Geometry: final body of the model. Coordinates: model frame, mm. A direction names the side the tool comes from. Coordinates: 2 decimals unless noted, no trailing zeros. Write each loop counter-clockwise with the first axis right and the second up, starting at its lowest first coordinate (ties: lowest second). Pieces come first, ordered by that corner, then holes. Notation, with made-up numbers: M -2.5,13.25 L 1.5,13.25 A21 cw 1.5,48.25 Z; hole C 49,30.25 d7. An arc over 180 degrees is marked long. Write item = value, one per line. Start each with the question number.
Item 1: Section C-C on x = 15.5. Output: boundary loops of the cut face in (y, z) (1 decimal).
Item 2: Section A-A on x = 0. Output: boundary loops of the cut face in (y, z).
Item 3: Pull-direction query (Y, two-part tool) for faces 1 (the cylindrical face through (19.492, 1.086, 0.236)), 2 (the flat face through (17, 16, 12.763)), 3 (the cylindrical face through (-19.55, 21.2, 19.49)); classes: +Y half, -Y half, draft (parallel to the pull), parting line (faces both ways), or undercut.
Item 4: First-contact query: pin 1 Ø2.5 at (x, z) = (1.5, 17) entering from +Y; pin 2 Ø13 at (x, z) = (-0.5, -1.5) entering from +Y. Flat tips, straight axial feed; report the tip coordinate or a pass-through.
Item 5: Section D-D on y = 7.5. Output: boundary loops of the cut face in (x, z), plus the area to 3 significant figures.
Item 6: Section B-B on z = 0. Output: boundary loops of the cut face in (x, y).
Item 7: Ray query, L1, parallel to Z at x = -16.5, y = 27; L2, parallel to X at y = 20, z = -14.5; L3, parallel to Z at x = 0, y = 1.95. Return the intervals inside material, ascending. Write a range as [from, to].
Item 8: Reachability of faces 4 (the cylindrical face through (-19.492, 1.086, -0.236)), 5 (the cylindrical face through (17.6, 35.9, -10.2)), 6 (the flat face through (0, 12.7, 17)) from +Z, -Z, +X, -X, +Y, -Y: full face, straight path, thin tool, end or side. Return the list, or none.
from build123d import *

# Parameters (mm, degrees)
SKETCH1_W           = 26.035
SKETCH1_H           = 26.035
SKETCH1_R           = 1.778
BOSS_EXTRUDE1_DEPTH = 5.08
SKETCH9_W           = 41.275
SKETCH9_H           = 41.275
SKETCH9_W_2         = 26.035
SKETCH9_H_2         = 26.035
BOSS_EXTRUDE7_DEPTH = 38.1
CUT_EXTRUDE4_DEPTH  = 42.275
SKETCH11_R          = 3.048
CUT_EXTRUDE5_DEPTH  = 42.275
FILLET1_R           = 3.81
FILLET2_R           = 3.81
SKETCH12_R          = 5.461
SKETCH12_R_2        = 3.048
CUT_EXTRUDE6_DEPTH  = 6.096
CUT_EXTRUDE7_START  = -41.275
SKETCH12_3_R        = 5.461
CUT_EXTRUDE7_DEPTH  = 6.096
SKETCH13_W          = 25.4
SKETCH13_H          = 12.7
CUT_EXTRUDE8_DEPTH  = 42.275
FILLET3_R           = 3.81
FILLET4_R           = 3.81


with BuildPart() as part:
    # Sketch1 → Boss-Extrude1 (new body)
    with BuildSketch(Plane(origin=(0, 0, 0), x_dir=(1, 0, 0), z_dir=(0, 1, 0))):
        Rectangle(SKETCH1_W, SKETCH1_H)
        with Locations((0, 9.525)):
            Circle(SKETCH1_R, mode=Mode.SUBTRACT)
        with Locations((-9.525, 0)):
            Circle(SKETCH1_R, mode=Mode.SUBTRACT)
        with Locations((9.525, 0)):
            Circle(SKETCH1_R, mode=Mode.SUBTRACT)
        with Locations((0, -9.525)):
            Circle(SKETCH1_R, mode=Mode.SUBTRACT)
    extrude(amount=BOSS_EXTRUDE1_DEPTH)

    # Sketch9 → Boss-Extrude7 (add)
    with BuildSketch(Plane.XZ):
        Rectangle(SKETCH9_W, SKETCH9_H)
        Rectangle(SKETCH9_W_2, SKETCH9_H_2, mode=Mode.SUBTRACT)
    extrude(amount=-BOSS_EXTRUDE7_DEPTH)

    # Sketch10 → Cut-Extrude4 (cut, through all)
    with BuildSketch(Plane.XY.offset(20.6375)):
        with BuildLine():
            Line((-13.0175, 20.32), (-13.0175, 38.1))
            Line((-13.0175, 38.1), (13.0175, 38.1))
            Line((13.0175, 38.1), (13.0175, 20.32))
            ThreePointArc((13.0175, 20.32), (10.785653673, 14.931846327), (5.3975, 12.7))
            Line((5.3975, 12.7), (-5.3975, 12.7))
            ThreePointArc((-5.3975, 12.7), (-10.785653673, 14.931846327), (-13.0175, 20.32))
        make_face()
    extrude(amount=-CUT_EXTRUDE4_DEPTH, mode=Mode.SUBTRACT)

    # Sketch11 → Cut-Extrude5 (cut, through all)
    with BuildSketch(Plane.ZY.offset(20.6375)):
        with Locations((-9.525, 30.48)):
            Circle(SKETCH11_R)
        with Locations((9.525, 30.48)):
            Circle(SKETCH11_R)
    extrude(amount=-CUT_EXTRUDE5_DEPTH, mode=Mode.SUBTRACT)

    # Fillet1
    fillet1_edges = [part.edges().sort_by_distance(p)[0] for p in [
        (20.6375, 19.05, -20.6375),
        (-20.6375, 19.05, -20.6375),
        (-20.6375, 19.05, 20.6375),
        (20.6375, 19.05, 20.6375),
    ]]
    fillet(fillet1_edges, radius=FILLET1_R)

    # Fillet2
    fillet2_edges = [part.edges().sort_by_distance(p)[0] for p in [
        (0, 0, -20.6375),
        (20.6375, 0, 0),
        (0, 0, 20.6375),
        (-20.6375, 0, 0),
        (-19.521576836, 0, 19.521576836),
        (-19.521576836, 0, -19.521576836),
        (19.521576836, 0, 19.521576836),
        (19.521576836, 0, -19.521576836),
    ]]
    fillet(fillet2_edges, radius=FILLET2_R)

    # Sketch12 → Cut-Extrude6 (cut)
    with BuildSketch(Plane.ZY.offset(20.6375)):
        with Locations((-9.525, 30.48)):
            Circle(SKETCH12_R)
        with Locations((-9.525, 30.48)):
            Circle(SKETCH12_R_2, mode=Mode.SUBTRACT)
        with Locations((9.525, 30.48)):
            Circle(SKETCH12_R)
        with Locations((9.525, 30.48)):
            Circle(SKETCH12_R_2, mode=Mode.SUBTRACT)
    extrude(amount=-CUT_EXTRUDE6_DEPTH, mode=Mode.SUBTRACT)

    # Sketch12<3> → Cut-Extrude7 (cut)
    with BuildSketch(Plane.ZY.offset(20.6375).offset(CUT_EXTRUDE7_START)):
        with Locations((-9.525, 30.48)):
            Circle(SKETCH12_3_R)
        with Locations((9.525, 30.48)):
            Circle(SKETCH12_3_R)
    extrude(amount=CUT_EXTRUDE7_DEPTH, mode=Mode.SUBTRACT)

    # Sketch13 → Cut-Extrude8 (cut, through all)
    with BuildSketch(Plane.ZY.offset(20.6375)):
        with Locations((0.0635, 15.748)):
            Rectangle(SKETCH13_W, SKETCH13_H)
    extrude(amount=-CUT_EXTRUDE8_DEPTH, mode=Mode.SUBTRACT)

    # Fillet3
    fillet3_edges = [part.edges().sort_by_distance(p)[0] for p in [
        (-20.6375, 9.398, 0.0635),
    ]]
    fillet(fillet3_edges, radius=FILLET3_R)

    # Fillet4
    fillet4_edges = [part.edges().sort_by_distance(p)[0] for p in [
        (20.6375, 9.398, 0.0635),
    ]]
    fillet(fillet4_edges, radius=FILLET4_R)


solid = part.part
Responses:
q1.outline = M 0,-16.8 A3.8 ccw 3.8,-20.6 L 38.1,-20.6 L 38.1,20.6 L 3.8,20.6 A3.8 ccw 0,16.8 Z; hole M 9.4,-12.6 L 22.1,-12.6 L 22.1,12.8 L 9.4,12.8 Z; hole C 30.5,-9.5 d10.9; hole C 30.5,9.5 d10.9
q2.outline = M 0,-16.83 A3.81 ccw 3.81,-20.64 L 12.7,-20.64 L 12.7,-13.02 L 5.08,-13.02 L 5.08,-11.3 L 0,-11.3 Z; M 0,-7.75 L 5.08,-7.75 L 5.08,7.75 L 0,7.75 Z; M 0,11.3 L 5.08,11.3 L 5.08,13.02 L 12.7,13.02 L 12.7,20.64 L 3.81,20.64 A3.81 ccw 0,16.83 Z
q3.face_1 = -Y half
q3.face_2 = undercut
q3.face_3 = draft
q4.pin_1 = 12.7
q4.pin_2 = 5.08
q5.outline = M -20.64,-16.83 A3.81 ccw -16.83,-20.64 L 16.83,-20.64 A3.81 ccw 20.64,-16.83 L 20.64,-12.64 L 20.12,-12.64 L 20.12,12.76 L 20.64,12.76 L 20.64,16.83 A3.81 ccw 16.83,20.64 L -16.83,20.64 A3.81 ccw -20.64,16.83 L -20.64,12.76 L -20.12,12.76 L -20.12,-12.64 L -20.64,-12.64 Z; hole M -13.02,-13.02 L 13.02,-13.02 L 13.02,13.02 L -13.02,13.02 Z
q5.area = 987 mm²
q6.outline = M -20.64,3.81 A3.81 ccw -16.83,0 L -11.3,0 L -11.3,5.08 L -13.02,5.08 L -13.02,9.4 L -16.83,9.4 A3.81 ccw -20.64,5.59 Z; M -20.64,22.1 L -13.02,22.1 L -13.02,38.1 L -20.64,38.1 Z; M -7.75,0 L 7.75,0 L 7.75,5.08 L -7.75,5.08 Z; M 11.3,0 L 16.83,0 A3.81 ccw 20.64,3.81 L 20.64,5.59 A3.81 ccw 16.83,9.4 L 13.02,9.4 L 13.02,5.08 L 11.3,5.08 Z; M 13.02,22.1 L 20.64,22.1 L 20.64,38.1 L 13.02,38.1 Z
q7.L1 = [-20.64, -13.73], [-5.32, 5.32], [13.73, 20.64]
q7.L2 = [-20.64, -13.01], [13.01, 20.64]
q7.L3 = [-20.15, -11.3], [-7.75, 7.75], [11.3, 20.15]
q8.face_4 = +Z, -Z, -X, -Y
q8.face_5 = +X
q8.face_6 = +Z, -Z, +Y
